Geometry check sheet. Reference: the model listing, model coordinates, mm. A direction names the side the tool comes from. Give positions to 0.01 mm unless a question says otherwise; leave off trailing zeros. Loops run counter-clockwise (first coordinate to the right, second up) from the corner with the lowest first, then second, coordinate; pieces in that order, holes last. Notation, with made-up numbers: (-2, -0.75) -> (4, -0.75) arc R23 cw to (4, 22.25) -> close; hole circle Ø10 at (-15, 80). An arc over 180 degrees is marked (long way). Write item = value, one per line.
```python
from build123d import *

# Parameters (mm, degrees)
F0_W     = 116.5
F0_H     = 116.5
F0_W_2   = 109.5
F0_H_2   = 109.5
F1_DEPTH = 136
F2_W     = 99.5149090886
F2_H     = 117.4702011049
F3_DEPTH = 186
F4_W     = 117.4702011049
F4_H     = 99.5149090886
F5_DEPTH = 134.2


# Not quite as in the source:
# - a feature of the source that left no trace in its solid (it failed there, or was rolled back) is left out


with BuildPart() as f1:
    # F0 (on Front) → F1 (new body)
    with BuildSketch(Plane.XZ):
        Rectangle(F0_W, F0_H)
        Rectangle(F0_W_2, F0_H_2, mode=Mode.SUBTRACT)
    extrude(amount=F1_DEPTH)

    # F2 (on face) → F3 (cut)
    with BuildSketch(Plane(origin=(0, 0, -58.25), x_dir=(1, 0, 0), z_dir=(0, 0, -1))):
        with Locations((0, 68.3887079358)):
            Rectangle(F2_W, F2_H)
    extrude(amount=-F3_DEPTH, mode=Mode.SUBTRACT)

    # F4 (on face) → F5 (cut)
    with BuildSketch(Plane.YZ.offset(58.25)):
        with Locations((-66.9774990529, -0.0578425825)):
            Rectangle(F4_W, F4_H)
    extrude(amount=-F5_DEPTH, mode=Mode.SUBTRACT)


solid = f1.part
```
Item 1: Section check C-C, the plane x = -24.5. Record the cut outline in (y, z).
Answer:
outline = (-136, -58.25) -> (-127.12, -58.25) -> (-127.12, -54.75) -> (-136, -54.75) -> close; (-136, 54.75) -> (-127.12, 54.75) -> (-127.12, 58.25) -> (-136, 58.25) -> close; (-9.65, -58.25) -> (0, -58.25) -> (0, -54.75) -> (-9.65, -54.75) -> close; (-9.65, 54.75) -> (0, 54.75) -> (0, 58.25) -> (-9.65, 58.25) -> close
Item 2: Section check B-B, the plane z = -31. Record the cut outline in (x, y), plus the area to 3 significant figures.
Answer:
outline = (-58.25, -136) -> (-54.75, -136) -> (-54.75, -125.71) -> (-58.25, -125.71) -> close; (-58.25, -8.24) -> (-54.75, -8.24) -> (-54.75, 0) -> (-58.25, 0) -> close; (54.75, -136) -> (58.25, -136) -> (58.25, -125.71) -> (54.75, -125.71) -> close; (54.75, -8.24) -> (58.25, -8.24) -> (58.25, 0) -> (54.75, 0) -> close
area = 130 mm^2
Item 3: Tool access check on faces 1 (the flat face through (-56, -125.713, -1)), 2 (the flat face through (-53, -73, -54.75)), 3 (the flat face through (-49.757, -68, 56)). Record the directions out of +Z, -Z, +X, -X, +Y, -Y that give a thin tool (end or side, any length) a straight path to the whole face; none if there is none.
Answer:
face_1 = +X, -X
face_2 = +Y, -Y
face_3 = +Z, -Z
Item 4: Thickness scan on L1, parallel to X at y = -39.5, z = 52. Record the ranges inside material, lowest first. Write a range as [from, to].
Answer:
L1 = [-58.25, -54.75], [54.75, 58.25]
Item 5: Draft check along X on faces 4 (the flat face through (-58.25, -67, 51)), 5 (the flat face through (-53, -73, 54.75)), 6 (the flat face through (51, -67, 58.25)), 7 (the flat face through (-54.75, -73, -53)). Enter one of: +X half, -X half, draft (parallel to the pull), parting line (faces both ways), or undercut.
Answer:
face_4 = -X half
face_5 = undercut
face_6 = draft
face_7 = undercut
Item 6: Section check A-A, the plane y = -109. Record the cut outline in (x, z).
Answer:
outline = (-58.25, -58.25) -> (-49.76, -58.25) -> (-49.76, -54.75) -> (-54.75, -54.75) -> (-54.75, -49.82) -> (-58.25, -49.82) -> close; (-58.25, 49.7) -> (-54.75, 49.7) -> (-54.75, 54.75) -> (-49.76, 54.75) -> (-49.76, 58.25) -> (-58.25, 58.25) -> close; (49.76, -58.25) -> (58.25, -58.25) -> (58.25, -49.82) -> (54.75, -49.82) -> (54.75, -54.75) -> (49.76, -54.75) -> close; (49.76, 54.75) -> (54.75, 54.75) -> (54.75, 49.7) -> (58.25, 49.7) -> (58.25, 58.25) -> (49.76, 58.25) -> close
Item 7: Gauge pin test, flat end, axial feed: pin 1 (6 mm diameter, centred on x = 44, y = -36, fed in from -Z). Record the tip position at first contact, or that the pin passes through.
Answer:
pin_1 = through
